Verification items for this drawing (mm, ordinates from the low corner). Round coordinates to 2 decimals unless told otherwise and drop trailing zeros. Write each loop counter-clockwise with the first axis right and the second up, starting at its lowest first coordinate (ties: lowest second). Pieces come first, ordered by that corner, then holes. Notation, with made-up numbers: (81.5, 14) -> (125.5, 14) arc R11 ccw to (125.5, 21) -> close; hole circle Ø6 at (34.25, -21). An arc over 180 degrees is marked (long way). One line per question, with ' | ' between items.
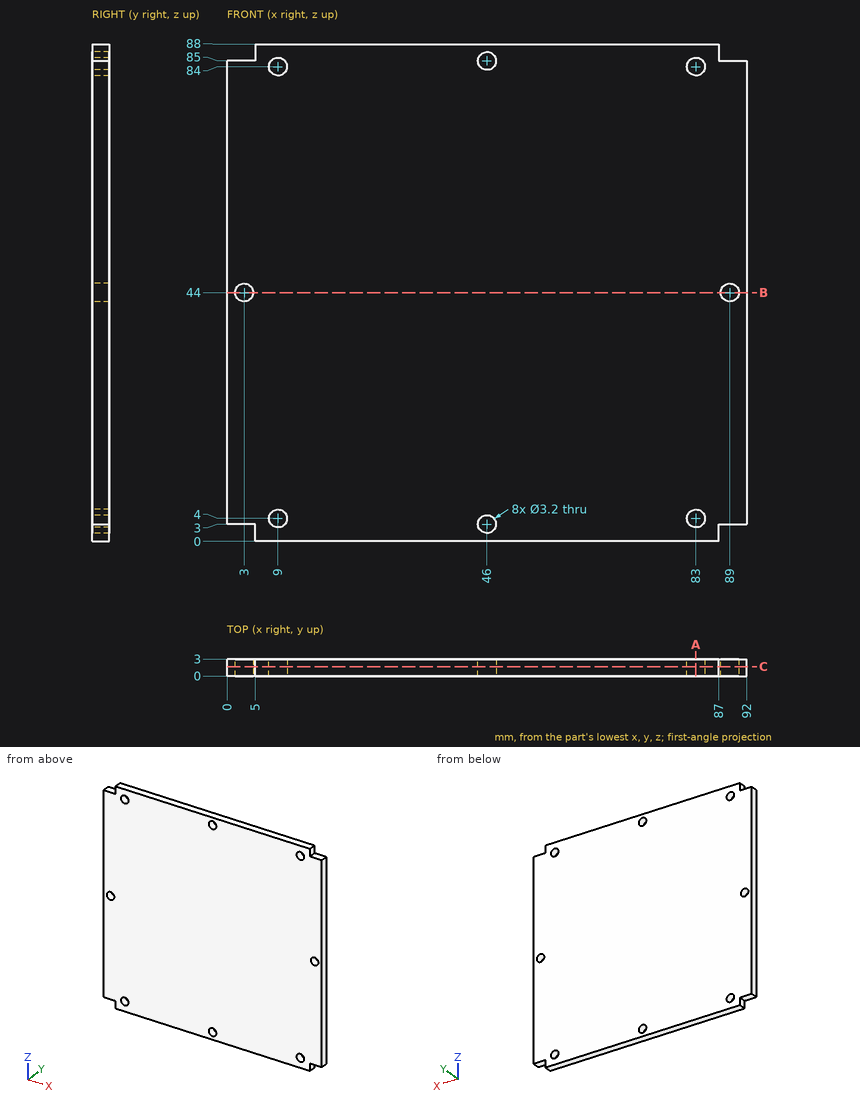
(1) Sectioned sample at C-C on y = 1.65. Count the separate pieces of the cut face and the enclosed holes in it, then the cut area to 3 significant figures.
Resolved:
separate pieces: 1 | enclosed holes: 8 | area: 7,970 mm2
(2) Material ranges on line 1 (Z direction, x = 83, y = 2.2); line 2 (Z direction, x = 46, y = 2.1); line 3 (Z direction, x = 3, y = 0.8), recorded low to high.
Resolved:
line 1: z = 0 to 2.4, 5.6 to 82.4, 85.6 to 88 | line 2: z = 0 to 1.4, 4.6 to 83.4, 86.6 to 88 | line 3: z = 3 to 42.4, 45.6 to 85
(3) Sectioned sample at A-A on x = 83. Record the cut outline in (y, z).
Resolved:
outline: (0, 0) -> (3, 0) -> (3, 2.4) -> (0, 2.4) -> close; (0, 5.6) -> (3, 5.6) -> (3, 82.4) -> (0, 82.4) -> close; (0, 85.6) -> (3, 85.6) -> (3, 88) -> (0, 88) -> close
(4) Sectioned sample at B-B on z = 44. Record the cut outline in (x, y).
Resolved:
outline: (0, 0) -> (1.4, 0) -> (1.4, 3) -> (0, 3) -> close; (4.6, 0) -> (87.4, 0) -> (87.4, 3) -> (4.6, 3) -> close; (90.6, 0) -> (92, 0) -> (92, 3) -> (90.6, 3) -> close
(5) Go/stop test with flat-tipped pins: pin 1 (2.5 mm diameter, centred on x = 3, z = 44, fed in from +Y); pin 2 (0.9 mm diameter, centred on y = 1, z = 86, fed in from +X); pin 3 (1.5 mm diameter, centred on x = 89, y = 1, fed in from -Z); pin 4 (0.9 mm diameter, centred on x = 90, y = 1.5, fed in from +Z). Record where each tip stops, or that it passes through.
Resolved:
pin 1: passes through | pin 2: stops at x = 87 | pin 3: stops at z = 3 | pin 4: stops at z = 85
